from build123d import *

# Parameters (mm, degrees)
SKETCH3_R          = 7.2
CUT_EXTRUDE1_DEPTH = 11.312366363
SKETCH4_R          = 3.5
CUT_EXTRUDE2_DEPTH = 5.14
SKETCH5_R          = 0.925
CUT_EXTRUDE3_DEPTH = 12.956372442


with BuildPart() as part:
    # Sketch1 → Revolve1 (revolve)
    with BuildSketch(Plane.XY, mode=Mode.PRIVATE) as revolve1_sk:
        Polygon((0, 7.3), (0, 0), (1.97, 0), (1.97, 0.9), (5.17, 0.9), (5.17, 0.4), (6.7, 0.4), (6.7, 3.23), (5.17, 3.23), (5.17, 2.16), (3, 2.16), (3, 7.3), align=None)
    revolve(revolve1_sk.sketch.rotate(Axis((0, 7.3, 0), (0, -1, 0)), 90), axis=Axis((0, 7.3, 0), (0, -1, 0)))

    # Sketch3 → Cut-Extrude1 (cut, through all)
    with BuildSketch(Plane(origin=(0, 3.23, 0), x_dir=(1, 0, 0), z_dir=(0, 1, 0))):
        Circle(SKETCH3_R)
        Polygon((0, 6.7), (-0.599928149, 5.899575088), (-1.348700085, 6.562850606), (-1.775223319, 5.65804579), (-2.642184229, 6.157017338), (-2.877840638, 5.184875434), (-3.827497041, 5.499115056), (-3.862638823, 4.499435668), (-4.856111674, 4.616078358), (-4.68930012, 3.629788477), (-5.685916525, 3.544058869), (-5.32398092, 2.611537319), (-6.282939285, 2.326945194), (-5.740697315, 1.486369516), (-6.622737773, 1.014566109), (-5.922388888, 0.300349571), (-6.691400598, -0.339349431), (-5.861617163, -0.897966721), (-6.486116696, -1.679371966), (-5.560870144, -2.059520149), (-6.015290415, -2.950640815), (-5.032460447, -3.136756581), (-5.298197437, -4.101110083), (-4.298021228, -4.08557383), (-4.364195634, -5.083679422), (-3.387620516, -4.867127206), (-3.251523149, -5.858122328), (-2.338530221, -5.449419823), (-2.005732924, -6.392733018), (-1.193700224, -5.808612552), (-0.677827757, -6.665624467), (0, -5.93), (0.677827757, -6.665624467), (1.193700224, -5.808612552), (2.005732924, -6.392733018), (2.338530221, -5.449419823), (3.251523149, -5.858122328), (3.387620516, -4.867127206), (4.364195634, -5.083679422), (4.298021228, -4.08557383), (5.298197437, -4.101110083), (5.032460447, -3.136756581), (6.015290415, -2.950640815), (5.560870144, -2.059520149), (6.486116696, -1.679371966), (5.861617163, -0.897966721), (6.691400598, -0.339349431), (5.922388888, 0.300349571), (6.622737773, 1.014566109), (5.740697315, 1.486369516), (6.282939285, 2.326945194), (5.32398092, 2.611537319), (5.685916525, 3.544058869), (4.68930012, 3.629788477), (4.856111674, 4.616078358), (3.862638823, 4.499435668), (3.827497041, 5.499115056), (2.877840638, 5.184875434), (2.642184229, 6.157017338), (1.775223319, 5.65804579), (1.348700085, 6.562850606), (0.599928149, 5.899575088), align=None, mode=Mode.SUBTRACT)
    extrude(amount=-CUT_EXTRUDE1_DEPTH, mode=Mode.SUBTRACT)

    # Sketch4 → Cut-Extrude2 (cut)
    with BuildSketch(Plane(origin=(0, 7.3, 0), x_dir=(1, 0, 0), z_dir=(0, 1, 0))):
        Circle(SKETCH4_R)
        Polygon((0, 3), (-0.684040287, 1.879385242), (-1.928362829, 2.298133329), (-1.732050808, 1), (-2.954423259, 0.520944533), (-1.969615506, -0.347296355), (-2.598076211, -1.5), (-1.285575219, -1.532088886), (-1.02606043, -2.819077862), (0, -2), (1.02606043, -2.819077862), (1.285575219, -1.532088886), (2.598076211, -1.5), (1.969615506, -0.347296355), (2.954423259, 0.520944533), (1.732050808, 1), (1.928362829, 2.298133329), (0.684040287, 1.879385242), align=None, mode=Mode.SUBTRACT)
    extrude(amount=-CUT_EXTRUDE2_DEPTH, mode=Mode.SUBTRACT)

    # Sketch5 → Cut-Extrude3 (cut, through all)
    with BuildSketch(Plane(origin=(0, 7.3, 0), x_dir=(1, 0, 0), z_dir=(0, 1, 0))):
        with Locations(Location((0, 0, 0), (0, 0, 270))):
            Circle(SKETCH5_R)
    extrude(amount=-CUT_EXTRUDE3_DEPTH, mode=Mode.SUBTRACT)


solid = part.part
The listing builds one solid part. Answer for the finished solid, in the listing's coordinates (mm). A direction names the side the tool comes from. Give positions to 0.01 mm unless a question says otherwise; leave off trailing zeros. Order: outer loops, then holes, each group sorted by start corner. A loop starts at its lowest first (then second) coordinate and runs counter-clockwise, first axis right, second up. Notation, with made-up numbers: (-30.5, -26.75) - (-14.5, -26.75) arc R26 ccw to (-14.5, -6.75) - close; hole circle Ø5 at (88.25, 84.5). An arc over 180 degrees is marked (long way). Use one line per item in the form item = value.
1) Find section A-A on z = 0. Determine the outline of the cut face in (x, y) (3 decimals), and give its area (3 significant figures).
Verdict:
outline = (-6.283, 0.4) - (-5.17, 0.4) - (-5.17, 0.9) - (-1.97, 0.9) - (-1.97, 0) - (-0.925, 0) - (-0.925, 7.3) - (-2.364, 7.3) - (-2.364, 2.16) - (-5.17, 2.16) - (-5.17, 3.23) - (-6.283, 3.23) - close; (0.925, 0) - (1.97, 0) - (1.97, 0.9) - (5.17, 0.9) - (5.17, 0.4) - (6.283, 0.4) - (6.283, 3.23) - (5.17, 3.23) - (5.17, 2.16) - (2.364, 2.16) - (2.364, 7.3) - (0.925, 7.3) - close
area = 33.7 mm^2
2) For faces 4 (the flat face through (-1.6, 1.8, 6.1)), 5 (the flat face through (5.517, 1.835, 3.045)), 6 (the flat face through (2.352, 4.766, -0.757)), 7 (the flat face through (-2.758, 1.835, -5.678)), determine the directions among +Z, -Z, +X, -X, +Y, -Y from which every point of the face is accessible in a straight line to the end or side of a thin tool.
Verdict:
face_4 = +Z, +Y, -Y
face_5 = +X, +Y, -Y
face_6 = +Y
face_7 = -Z, +Y, -Y
3) The mould has two halves that part along Z. Classify faces 1 (the flat face through (2.17, 1.83, 5.93)), 2 (the flat face through (-6.18, 1.83, -1.25)), 3 (the flat face through (4.37, 1.83, -4.56)): released by +Z, released by -Z, zero draft, split by the parting line, or undercut.
Verdict:
face_1 = released by +Z
face_2 = undercut
face_3 = released by -Z
4) This flat-tipped pin is pushed along its axis until it touches: pin 1 (1 mm diameter, centred on y = 2.5, z = -5, fed in from -X). Where does it stop, or does it pass through?
Verdict:
pin_1 = -4.86
5) Consider probe 1 along X at (y, z) = (0.75, 0) (3 decimals); probe 2 along X at (y, z) = (3, 1.75); probe 3 along Y at (x, z) = (5.5, -3.5). Determine where each line is inside the solid, lowest interval first. Write a range as [from, to].
Verdict:
probe_1 = [-6.283, -5.17], [-1.97, -0.925], [0.925, 1.97], [5.17, 6.283]
probe_2 = [-6.31, -4.86], [-1.24, 1.24], [4.86, 6.31]
probe_3 = [0.4, 3.23]
